Here's how the part is built. I have some questions about the finished solid (model axes, mm). Coordinates: 2 decimals unless noted, no trailing zeros. Loops run counter-clockwise (first coordinate to the right, second up) from the corner with the lowest first, then second, coordinate; pieces in that order, holes last.
```python
from build123d import *

# Parameters (mm, degrees)
BASPROSKE_W         = 5.842
BASPROSKE_H         = 19.05
TOOTHCUT_DEPTH      = 28.566899789
TEETHCUTS_COUNT     = 10
TEETHCUTS_ANGLE     = 324
BORSKE_R            = 2.38125
BORE_DEPTH          = 50.8000508
BOSS_EXTRUDE1_DEPTH = 5.842
BOSS_EXTRUDE2_DEPTH = 5.842


with BuildPart() as part:
    # BasProSke → Base-Revolve (revolve)
    with BuildSketch(Plane(origin=(0, 0, 0), x_dir=(1, 0, 0), z_dir=(0, 1, 0)), mode=Mode.PRIVATE) as base_revolve_sk:
        with Locations((2.921, 9.525)):
            Rectangle(BASPROSKE_W, BASPROSKE_H)
    revolve(base_revolve_sk.sketch.rotate(Axis((-10, 0, 0), (1, 0, 0)), 180), axis=Axis((-10, 0, 0), (1, 0, 0)))

    # TooCutSke → ToothCut (cut, through all)
    with BuildSketch(Plane(origin=(0, 0, 0), x_dir=(0, 0, -1), z_dir=(1, 0, 0))):
        with BuildLine():
            ThreePointArc((1.873548596, 11.756630659), (0, 11.90498), (-1.873548596, 11.756630659))
            ThreePointArc((-1.873548596, 11.756630659), (-2.656568084, 15.60034376), (-5.548507123, 18.250615164))
            ThreePointArc((-5.548507123, 18.250615164), (0, 19.0754), (5.548507123, 18.250615164))
            ThreePointArc((5.548507123, 18.250615164), (2.656568084, 15.60034376), (1.873548596, 11.756630659))
        make_face()
    toothcut = extrude(amount=TOOTHCUT_DEPTH, mode=Mode.SUBTRACT)

    # TeethCuts: ToothCut ×10 about axis
    teethcuts_axis = Axis((-10, 0, 0), (1, 0, 0))
    for i in range(1, TEETHCUTS_COUNT):
        add(toothcut.rotate(teethcuts_axis, i * TEETHCUTS_ANGLE / (TEETHCUTS_COUNT - 1)), mode=Mode.SUBTRACT)

    # BorSke → Bore (cut, symmetric)
    with BuildSketch(Plane(origin=(0, 0, 0), x_dir=(0, 0, -1), z_dir=(1, 0, 0))):
        with Locations(Location((0, 0, 0), (0, 0, 180))):
            Circle(BORSKE_R)
    extrude(amount=BORE_DEPTH, both=True, mode=Mode.SUBTRACT)

    # Sketch1 → Boss-Extrude1 (add)
    with BuildSketch(Plane(origin=(5.842, 0, 0), x_dir=(0, 0, -1), z_dir=(1, 0, 0))):
        with BuildLine():
            Line((-4.4067353, 4.572), (4.4067353, 4.572))
            ThreePointArc((4.4067353, 4.572), (0, 6.35), (-4.4067353, 4.572))
        make_face()
    extrude(amount=-BOSS_EXTRUDE1_DEPTH)

    # Sketch2 → Boss-Extrude2 (add)
    with BuildSketch(Plane(origin=(5.842, 0, 0), x_dir=(0, 0, -1), z_dir=(1, 0, 0))):
        with BuildLine():
            Line((-2.177028232, 1.27), (2.177028232, 1.27))
            ThreePointArc((2.177028232, 1.27), (0, 2.520387256), (-2.177028232, 1.27))
        make_face()
        with BuildLine():
            Line((-2.177028232, -1.27), (2.177028232, -1.27))
            ThreePointArc((2.177028232, -1.27), (0, -2.520387256), (-2.177028232, -1.27))
        make_face()
    extrude(amount=-BOSS_EXTRUDE2_DEPTH)


solid = part.part
```
1. I want a section at A-A (z = 14.5). Please give me the cut outline in (x, y), then the cut area to 3 significant figures.
2. We'd pull the mould along Y, two halves only. Please class faces 1 (the flat face through (0, 4, 0)), 2 (the cylindrical face through (2.88, -9.647, -6.976)): +Y half, -Y half, draft (parallel to the pull), parting line (faces both ways), or undercut.
3. For pin 1 (3 mm diameter, centred on x = 3, z = -10.5, fed in from -Y); pin 2 (1.2 mm diameter, centred on x = 2, z = 0, fed in from -Y) (3 decimals); pin 3 (1.2 mm diameter, centred on x = 3, z = -0.5, fed in from +Y) (3 decimals), each with a flat end and sliding along its axis, tell me the tip position at first contact or that it passes through.
4. I want a section at C-C (z = -1). Please give me the cut outline in (x, y).
5. I need wall thicknesses on line 1 along Z through (x, y) = (3.65, 0); line 2 along Y through (x, z) = (4.2, -0.5); line 3 along Y through (x, z) = (4.75, -6). Which ranges of each line are inside material? Lowest first, please.
6. I want a section at D-D (y = -4.5). Please give me the cut outline in (x, z), then the cut area to 3 significant figures.
7. I want a section at B-B (y = 9.5). Please give me the cut outline in (x, z).
Response values:
1. outline: (0, -11.61) - (5.84, -11.61) - (5.84, -7.94) - (0, -7.94) - close; (0, -2.42) - (5.84, -2.42) - (5.84, 2.42) - (0, 2.42) - close; (0, 7.94) - (5.84, 7.94) - (5.84, 11.61) - (0, 11.61) - close
1. area: 71.1 mm2
2. face 1: draft
2. face 2: undercut
3. pin 1: stops at y = -11.32
3. pin 2: stops at y = -11.905
3. pin 3: stops at y = 11.905
4. outline: (0, -11.86) - (5.84, -11.86) - (5.84, -1.27) - (0, -1.27) - close; (0, 1.27) - (5.84, 1.27) - (5.84, 11.86) - (0, 11.86) - close
5. line 1: z = -19.05 to -2.38, 2.38 to 19.05
5. line 2: y = -11.89 to -1.27, 1.27 to 11.89
5. line 3: y = -18.08 to -11.39, -10.28 to 10.28, 11.39 to 18.08
6. outline: (0, -11.02) - (5.84, -11.02) - (5.84, 11.02) - (0, 11.02) - close
6. area: 129 mm2
7. outline: (0, -15.31) - (5.84, -15.31) - (5.84, -9.21) - (0, -9.21) - close; (0, -7.17) - (5.84, -7.17) - (5.84, 7.17) - (0, 7.17) - close; (0, 9.21) - (5.84, 9.21) - (5.84, 15.31) - (0, 15.31) - close
